Could you check a few things on this model? Use its own coordinates, in mm. Face numbers are marked on the shaded views. A direction names the side the tool comes from. Give positions to 0.01 mm unless a question says otherwise; leave off trailing zeros. Loops run counter-clockwise (first coordinate to the right, second up) from the corner with the lowest first, then second, coordinate; pieces in that order, holes last.
1. For the marked faces 5, 6 and 7, which set-ups out of +Z, -Z, +X, -X, +Y, -Y let a thin tool reach every point of the face, with its end or its side?
2. Imagine slicing it at B-B (x = 33.5). List the corners of the cut face in (y, z) for me, plus the area to 3 significant figures.
3. Thinking about a two-plate mould opening in X: for the marked faces 1, 2, 3 and 4, which applies, +X half, -X half, draft (parallel to the pull), parting line (faces both ways), or undercut?
4. Imagine slicing it at C-C (x = 13). List the corners of the cut face in (y, z) for me, plus the area to 3 significant figures.
5. I need wall thicknesses on line 1 along X through (y, z) = (3, 2.5); line 2 along X through (y, z) = (-2, 0.5); line 3 along Y through (x, z) = (2, -7). Which ranges of each line are inside material? Lowest first, please.
6. Imagine slicing it at A-A (z = -15.5). List the corners of the cut face in (x, y) for me.
7. For P1, Ø10, axis at y = 14, z = -13, coming from the -X side; P2, Ø1.5, axis at y = 8.5, z = -9, coming from the +X side; P3, Ø10, axis at y = -0.5, z = -6, coming from the +X side; P4, Ø2, axis at y = -11.5, z = 0, coming from the +X side, each with a flat end and sliding along its axis, tell me the tip position at first contact or that it passes through.
```python
from build123d import *

# Parameters (mm, degrees)
SKETCH2_R           = 6
BOSS_EXTRUDE1_DEPTH = 6.5
SKETCH3_R           = 3
BOSS_EXTRUDE2_DEPTH = 15.5
CUT_EXTRUDE1_DEPTH  = 12
CHAMFER1_SIZE       = 1
SKETCH5_R           = 1.23
CUT_EXTRUDE2_DEPTH  = 5
CIRPATTERN1_COUNT   = 6
BOSS_EXTRUDE3_DEPTH = 7.9
BOSS_EXTRUDE4_DEPTH = 6.1
CHAMFER2_SIZE       = 0.5
BOSS_EXTRUDE5_DEPTH = 0.65
FILLET1_R           = 0.5
CUT_EXTRUDE3_DEPTH  = 1


with BuildPart() as part:
    # Sketch1 → Revolve1 (revolve)
    with BuildSketch(Plane.XY):
        with BuildLine():
            Line((0, 0), (64, 0))
            Line((64, 0), (64, 0.5))
            ThreePointArc((64, 0.5), (63.853553391, 0.853553391), (63.5, 1))
            Line((63.5, 1), (64, 1))
            Line((64, 1), (64, 5))
            Line((64, 5), (63.5, 5))
            Line((63.5, 5), (63.5, 9))
            Line((63.5, 9), (59, 9))
            Line((59, 9), (59, 1))
            Line((59, 1), (56.1, 1))
            Line((56.1, 1), (56.1, 13))
            Line((56.1, 13), (54.5, 13))
            Line((54.5, 13), (54.5, 1))
            Line((54.5, 1), (52, 1))
            Line((52, 1), (52, 17))
            Line((52, 17), (22, 17))
            Line((22, 17), (22, 18.4))
            Line((22, 18.4), (0, 18.4))
            Line((0, 18.4), (0, 0))
        make_face()
    revolve(axis=Axis((0, 0, 0), (1, 0, 0)))

    # Sketch2 → Boss-Extrude1 (add)
    with BuildSketch(Plane.ZY):
        with Locations((0, -7)):
            Circle(SKETCH2_R)
    extrude(amount=BOSS_EXTRUDE1_DEPTH)

    # Sketch3 → Boss-Extrude2 (add)
    with BuildSketch(Plane.ZY.offset(6.5)):
        with Locations((0, -7)):
            Circle(SKETCH3_R)
    extrude(amount=BOSS_EXTRUDE2_DEPTH)

    # Sketch4 → Cut-Extrude1 (cut)
    with BuildSketch(Plane.ZY.offset(22)):
        with BuildLine():
            Line((1.5, -9.598076211), (-1.5, -9.598076211))
            ThreePointArc((-1.5, -9.598076211), (0, -10), (1.5, -9.598076211))
        make_face()
    extrude(amount=-CUT_EXTRUDE1_DEPTH, mode=Mode.SUBTRACT)

    # Chamfer1
    chamfer1_edges = [part.edges().sort_by_distance(p)[0] for p in [
        (-6.5, -7, -6),
    ]]
    chamfer(chamfer1_edges, length=CHAMFER1_SIZE)

    # Sketch5 → Cut-Extrude2 (cut)
    with BuildSketch(Plane.ZY):
        with Locations((15.5, 0)):
            Circle(SKETCH5_R)
    cut_extrude2 = extrude(amount=-CUT_EXTRUDE2_DEPTH, mode=Mode.SUBTRACT)

    # CirPattern1: Cut-Extrude2 ×6 about axis
    cirpattern1_axis = Axis((0, 0, 0), (1, 0, 0))
    for i in range(1, CIRPATTERN1_COUNT):
        add(cut_extrude2.rotate(cirpattern1_axis, i * 360 / CIRPATTERN1_COUNT), mode=Mode.SUBTRACT)

    # Sketch6 → Boss-Extrude3 (add)
    with BuildSketch(Plane(origin=(56.1, 0, 0), x_dir=(0, 0, -1), z_dir=(1, 0, 0))):
        Polygon((0.614545099, 11.559081954), (5.734377326, 10.04515307), (5.196377764, 8.225736367), (0.076545537, 9.739665251), align=None)
    extrude(amount=BOSS_EXTRUDE3_DEPTH)

    # Sketch7 → Boss-Extrude4 (add)
    with BuildSketch(Plane(origin=(52, 0, 0), x_dir=(0, 0, -1), z_dir=(1, 0, 0))):
        Polygon((-10.569640254, 4.993749072), (-11.532445624, 1.431369202), (-10.567082231, 1.170460177), (-9.604276861, 4.732840047), align=None)
        Polygon((10.960206493, -0.825128427), (9.997401123, -4.387508297), (10.962764516, -4.648417322), (11.925569886, -1.086037452), align=None)
    extrude(amount=BOSS_EXTRUDE4_DEPTH)

    # Chamfer2
    chamfer2_edges = [part.edges().sort_by_distance(p)[0] for p in [
        (58.1, 1.300914689, 11.049763927),
        (58.1, 4.86329456, 10.086958557),
        (58.1, -4.51796281, -10.480082819),
        (58.1, -0.955582939, -11.44288819),
    ]]
    chamfer(chamfer2_edges, length=CHAMFER2_SIZE)

    # Sketch9 → Boss-Extrude5 (add)
    with BuildSketch(Plane(origin=(56.1, 0, 0), x_dir=(0, 0, -1), z_dir=(1, 0, 0))):
        Polygon((-7.807702145, -6.480963086), (-9.112247271, -11.307780051), (-8.484761066, -11.477370917), (-7.18021594, -6.650553952), align=None)
        Polygon((-5.932615753, -8.052596911), (-7.237160879, -12.879413876), (-6.609674674, -13.049004742), (-5.305129548, -8.222187777), align=None)
        Polygon((-3.769488931, -8.99589657), (-5.074034056, -13.822713535), (-4.446547851, -13.992304402), (-3.142002725, -9.165487437), align=None)
        Polygon((-1.65786261, -9.621868256), (-2.962407736, -14.448685221), (-2.33492153, -14.618276088), (-1.030376405, -9.791459122), align=None)
        Polygon((0.680101248, -9.624615249), (-0.624443878, -14.451432214), (0.003042327, -14.62102308), (1.307587453, -9.794206115), align=None)
        Polygon((2.920113487, -9.395250912), (1.615568361, -14.222067877), (2.243054567, -14.391658744), (3.547599693, -9.564841778), align=None)
    extrude(amount=BOSS_EXTRUDE5_DEPTH)

    # Fillet1
    fillet1_edges = [part.edges().sort_by_distance(p)[0] for p in [
        (56.75, -6.565758519, 7.493959043),
        (56.75, -8.137392344, 5.618872651),
        (56.75, -9.080692003, 3.455745828),
        (56.75, -9.706663689, 1.344119507),
        (56.75, -9.709410682, -0.99384435),
        (56.75, -9.480046345, -3.23385659),
    ]]
    fillet(fillet1_edges, radius=FILLET1_R)

    # Sketch14 → Cut-Extrude3 (cut)
    with BuildSketch(Plane.ZY):
        with BuildLine():
            ThreePointArc((-9.613871703, -7.181467181), (0, 12), (9.613871703, -7.181467181))
            ThreePointArc((9.613871703, -7.181467181), (8.626247239, -7.502469221), (7.993556247, -6.678972713))
            ThreePointArc((7.993556247, -6.678972713), (0, 1), (-7.993556247, -6.678972713))
            ThreePointArc((-7.993556247, -6.678972713), (-8.626247239, -7.502469221), (-9.613871703, -7.181467181))
        make_face()
    extrude(amount=-CUT_EXTRUDE3_DEPTH, mode=Mode.SUBTRACT)


solid = part.part
```
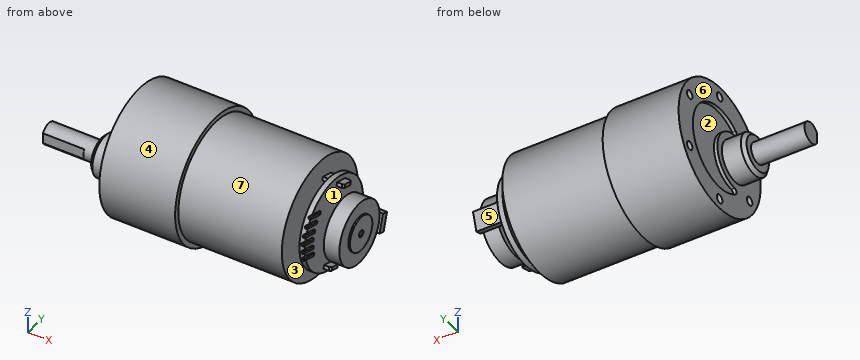
Derived:
1. face 5: -Z, +X, +Y
1. face 6: -X
1. face 7: +X
2. outline: circle Ø34 at (0, 0)
2. area: 908 mm2
3. face 1: undercut
3. face 2: -X half
3. face 3: undercut
3. face 4: draft
4. outline: circle Ø36.8 at (0, 0)
4. area: 1,060 mm2
5. line 1: x = 1 to 52, 54.5 to 56.1, 59 to 64
5. line 2: x = -6.48 to 52, 54.5 to 56.1, 59 to 64
5. line 3: y = -17.02 to -14.4, -12.45 to 12.45, 14.4 to 17.02
6. outline: (0, -9.92) - (22, -9.92) - (22, -6.98) - (52, -6.98) - (52, 6.98) - (22, 6.98) - (22, 9.92) - (0, 9.92) - (0, 1.23) - (5, 1.23) - (5, -1.23) - (0, -1.23) - close
7. P1: stops at x = 0
7. P2: stops at x = 56.1
7. P3: stops at x = 64
7. P4: stops at x = 56.75
